Could you check a few things on this model? Use its own coordinates, in mm. A direction names the side the tool comes from. Coordinates: 2 decimals unless noted, no trailing zeros. Order: outer loops, then holes, each group sorted by start corner. A loop starts at its lowest first (then second) coordinate and runs counter-clockwise, first axis right, second up. Notation, with made-up numbers: (85.25, 32) - (126.25, 32) arc R24 cw to (126.25, 59) - close; hole circle Ø5 at (88, 1.25). An arc over 180 degrees is marked (long way). Answer as CSV lines item,"result". Start each with the question number.
1. I want a section at A-A, the plane y = -1.1. List the corners of the cut face in (x, z) for me, and give its area (3 significant figures).
2. For faces 1 (the face through (3, 0, -7)), 2 (the face through (-6, 0, 5)), 3 (the face through (3, 0, 8)), which set-ups out of +Z, -Z, +X, -X, +Y, -Y let a thin tool reach every point of the face, with its end or its side?
3. I want a section at C-C, the plane x = -6.25. List the corners of the cut face in (y, z) for me, and give its area (3 significant figures).
4. I need wall thicknesses on probe 1 along Z at (x, y) = (-7.25, 0); probe 2 along X at (y, z) = (1.2, -4.75). Which ranges of each line are inside material? Lowest first, please.
5. For pin 1 (1.5 mm diameter, centred on y = -0.5, z = -4.5, fed in from +X); pin 2 (1.5 mm diameter, centred on y = 0, z = 7.5, fed in from +X); pin 3 (1.5 mm diameter, centred on y = 0.5, z = -7.5, fed in from -X), each with a flat end and sliding along its axis, tell me the tip position at first contact or that it passes through.
6. I want a section at B-B, the plane z = 7.25. List the corners of the cut face in (x, y) for me.
from build123d import *

# Parameters (mm, degrees)
SKETCH1_W           = 12
SKETCH1_H           = 12
BOSS_EXTRUDE1_DEPTH = 1.5
SKETCH2_W           = 6
SKETCH2_H           = 3
SKETCH2_W_2         = 3
SKETCH2_H_2         = 6
BOSS_EXTRUDE2_DEPTH = 1.5


with BuildPart() as part:
    # Sketch1 → Boss-Extrude1 (new body, symmetric)
    with BuildSketch(Plane(origin=(0, 0, 0), x_dir=(1, 0, 0), z_dir=(0, 1, 0))):
        Rectangle(SKETCH1_W, SKETCH1_H)
    extrude(amount=BOSS_EXTRUDE1_DEPTH, both=True)

    # Sketch2 → Boss-Extrude2 (add, symmetric)
    with BuildSketch(Plane(origin=(0, 0, 0), x_dir=(1, 0, 0), z_dir=(0, 1, 0))):
        with Locations((0, 7.5)):
            Rectangle(SKETCH2_W, SKETCH2_H)
        with Locations((0, -7.5)):
            Rectangle(SKETCH2_W, SKETCH2_H)
        with Locations((-7.5, 0)):
            Rectangle(SKETCH2_W_2, SKETCH2_H_2)
        with Locations((7.5, 0)):
            Rectangle(SKETCH2_W_2, SKETCH2_H_2)
    extrude(amount=BOSS_EXTRUDE2_DEPTH, both=True)


solid = part.part
Solved:
1,outline,"(-9, -3) - (-6, -3) - (-6, -6) - (-3, -6) - (-3, -9) - (3, -9) - (3, -6) - (6, -6) - (6, -3) - (9, -3) - (9, 3) - (6, 3) - (6, 6) - (3, 6) - (3, 9) - (-3, 9) - (-3, 6) - (-6, 6) - (-6, 3) - (-9, 3) - close"
1,area,"216 mm2"
2,face 1,"-Z, +X, +Y, -Y"
2,face 2,"+Z, -X, +Y, -Y"
2,face 3,"+Z, +X, +Y, -Y"
3,outline,"(-1.5, -3) - (1.5, -3) - (1.5, 3) - (-1.5, 3) - close"
3,area,"18.0 mm2"
4,probe 1,"z = -3 to 3"
4,probe 2,"x = -6 to 6"
5,pin 1,"stops at x = 6"
5,pin 2,"stops at x = 3"
5,pin 3,"stops at x = -3"
6,outline,"(-3, -1.5) - (3, -1.5) - (3, 1.5) - (-3, 1.5) - close"
